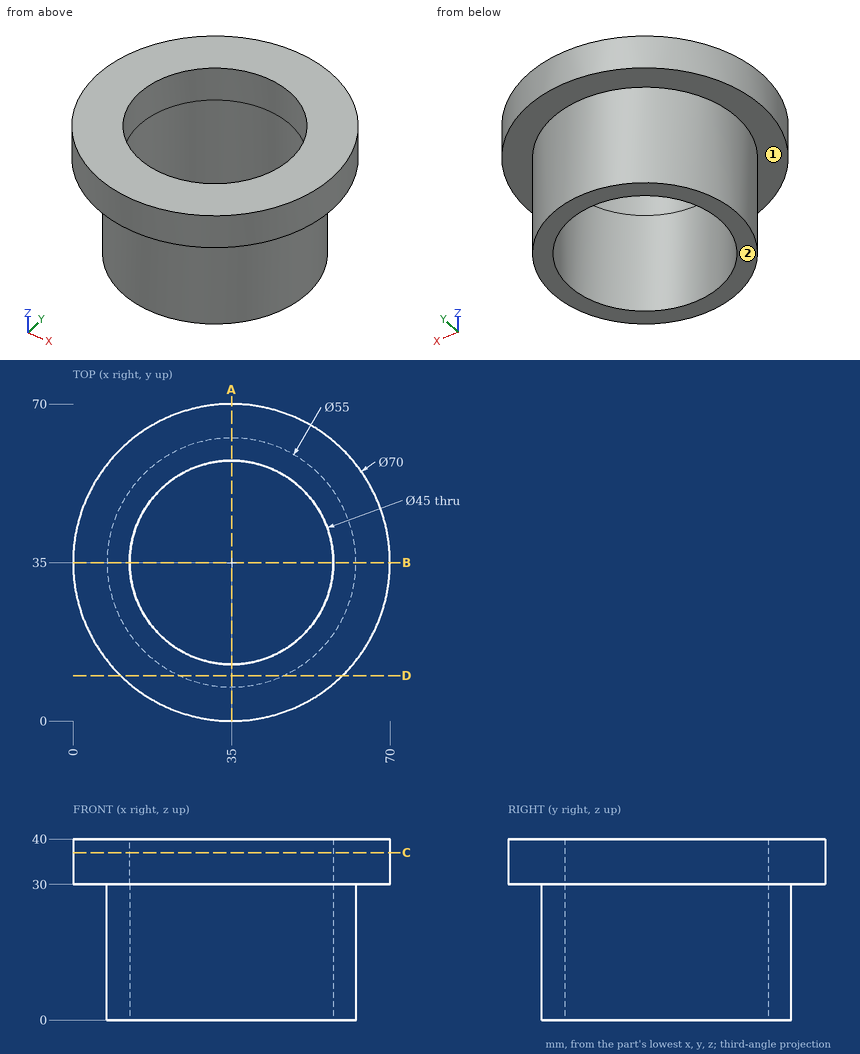
Print and shaded views of the part. All mm, measured from the part's lowest x, y and z. A direction names the side the tool comes from. Give positions to 0.01 mm unless a question says otherwise; leave off trailing zeros. Write each loop counter-clockwise with the first axis right and the second up, starting at its lowest first coordinate (ties: lowest second). Pieces come first, ordered by that corner, then holes. Notation, with made-up numbers: (32.25, 70) -> (82.25, 70) arc R21 cw to (82.25, 75) -> close; hole circle Ø8 at (-6.75, 1). An arc over 180 degrees is marked (long way). Write item = value, one per line.
(1) Probe line 1 along Y through (x, z) = (35, 9.75); line 2 along Y through (x, z) = (35, 32.5); line 3 along X through (y, z) = (18, 26.5). List the from-to ranges inside material, lowest first.
Determined:
line_1 = 7.5 to 12.5, 57.5 to 62.5
line_2 = 0 to 12.5, 57.5 to 70
line_3 = 13.38 to 20.26, 49.74 to 56.62
(2) Slice it at C-C, the plane z = 37. Give the cut face in (x, y).
Determined:
outline = circle Ø70 at (35, 35); hole circle Ø45 at (35, 35)
(3) Flat gauge pins, fed straight in: P1, Ø6, axis at y = 34, z = 32, coming from the -X side; P2, Ø4, axis at y = 26.5, z = 20.5, coming from the +X side; P3, Ø1, axis at y = 15, z = 24.5, coming from the -X side; P4, Ø12, axis at y = 59.5, z = 24.5, coming from the +X side. Where does each tip first touch, or does it go through?
Determined:
P1 = 0
P2 = 61.72
P3 = 15.61
P4 = 62.14
(4) Slice it at D-D, the plane y = 10. Give the cut face in (x, z), then the cut area to 3 significant figures.
Determined:
outline = (10.51, 30) -> (23.54, 30) -> (23.54, 0) -> (46.46, 0) -> (46.46, 30) -> (59.49, 30) -> (59.49, 40) -> (10.51, 40) -> close
area = 1,180 mm2
(5) Tool access for the marked faces 1 and 2: list every direction of +Z, -Z, +X, -X, +Y, -Y with a clear straight run to the whole face (end or side of a thin tool).
Determined:
face_1 = -Z
face_2 = -Z, +X, -X, +Y, -Y
(6) Slice it at A-A, the plane x = 35. Give the cut face in (y, z), then the cut area to 3 significant figures.
Determined:
outline = (0, 30) -> (7.5, 30) -> (7.5, 0) -> (12.5, 0) -> (12.5, 40) -> (0, 40) -> close; (57.5, 0) -> (62.5, 0) -> (62.5, 30) -> (70, 30) -> (70, 40) -> (57.5, 40) -> close
area = 550 mm2
